Autodesk Inventor part; units mm, degrees
ref_plane "YZ Plane" through (0, 0, 0) normal (1, 0, 0) x (0, 1, 0)
ref_plane "XZ Plane" through (0, 0, 0) normal (0, 1, 0) x (-1, 0, 0)
ref_plane "XY Plane" through (0, 0, 0) normal (0, 0, 1) x (1, 0, 0)
ref_plane "Work Plane1" through (0, 0, 0) normal (0, 0, 1) x (1, 0, 0)
sketch "Sketch1" plane through (0, 0, 0) normal (0, 0, 1) x (1, 0, 0)
  line L0 (21.3787, 6.8051) -> (32.3787, 6.8051)
  line L1 (32.3787, 6.8051) -> (32.3787, -2.1949)
  line L2 (32.3787, -2.1949) -> (21.3787, -2.1949)
  line L3 (21.3787, -2.1949) -> (21.3787, 6.8051)
  point P0 (0, 0)
  dimension "d0" = 11
  dimension "d2" = 9
extrude "Extrusion1" add sketch "Sketch1" along normal blind 5
sketch "Sketch2" plane through (32.3787, -2.1949, 0) normal (1, 0, 0) x (0, 0, -1)
  circle A0 centre (-2.5, 4.5) radius 3.1
  point P0 (0, 2.1949)
  dimension "d5" = 6.2
extrude "Extrusion2" add sketch "Sketch2" along normal blind 4
sketch "Sketch3" plane through (36.3787, 2.3051, 2.5) normal (1, 0, 0) x (0, 0, -1)
  circle A0 centre (0, 0) radius 3.1
  circle A1 centre (0, 0) radius 1.75
  point P0 (2.5, -2.3051)
  dimension "d9" = 3.5
extrude "Extrusion3" cut sketch "Sketch3" against normal blind 7 contours A1
properties part number "nanopc_t4_headphone"
Geometry: final body of the model. Coordinates: model frame, mm. A direction names the side the tool comes from. Round coordinates to 2 decimals unless told otherwise and drop trailing zeros. Write each loop counter-clockwise with the first axis right and the second up, starting at its lowest first coordinate (ties: lowest second). Pieces come first, ordered by that corner, then holes. Notation, with made-up numbers: M -29,28.5 L 2,28.5 A21 cw 2,32.5 Z; hole C 6.25,33.25 d3. An arc over 180 degrees is marked long. Answer in a Markdown table with one row per item. Add a question column.
(1) Cut plane D-D, the plane y = 0. Return the cut outline in (x, z), then the cut area to 3 significant figures.
(2) Reachability of faces 1 (the face through (36.379, 1, 1)), 2 (the face through (27, 2, 0)), 3 (the face through (32.928, 0.753, 1.692)) from +Z, -Z, +X, -X, +Y, -Y: full face, straight path, thin tool, end or side. Return the list, or none.
(3) Contact query for flat-ended pins moving along their axis: pin 1 (0.7 mm diameter, centred on y = 3, z = 5.5, fed in from -X); pin 2 (4 mm diameter, centred on x = 31, y = 0.5, fed in from +Z); pin 3 (1.5 mm diameter, centred on x = 33.5, z = 4.5, fed in from -Y). Output: stop coordinate, or through.
(4) Draft query along Y for faces 4 (the face through (34.351, 1.374, -0.457)), 5 (the face through (29.379, 2, 3)), 6 (the face through (27, 2, 5)). Return one class per face: pulls with the +Y half, pulls with the -Y half, needs draft (parallel to the pull), parting line crosses it, or undercut.
(5) Cut plane C-C, the plane x = 34.25. Return the cut outline in (y, z).
(6) Cut plane A-A, the plane z = 2.5. Return the cut outline in (x, y), then the cut area to 3 significant figures.
(7) Ray query, L1, parallel to Y at x = 32, z = 2.5; L2, parallel to Y at x = 33.5, z = 2.5; L3, parallel to Z at x = 24, y = 5. Return the intervals inside material, ascending.
(8) Cut plane B-B, the plane y = 1.25. Return the cut outline in (x, z), then the cut area to 3 significant figures.
Established:
| question | item | result |
|---|---|---|
| 1 | outline | M 21.38,0 L 32.38,0 L 32.38,0.43 L 36.38,0.43 L 36.38,4.57 L 32.38,4.57 L 32.38,5 L 21.38,5 Z |
| 1 | area | 71.6 mm² |
| 2 | face 1 | +Z, -Z, +X, +Y, -Y |
| 2 | face 2 | -Z, -X, +Y, -Y |
| 2 | face 3 | +X |
| 3 | pin 1 | x = 32.38 |
| 3 | pin 2 | z = 5.58 |
| 3 | pin 3 | y = -0.53 |
| 4 | face 4 | parting line crosses it |
| 4 | face 5 | undercut |
| 4 | face 6 | needs draft |
| 5 | outline | C 2.31,2.5 d6.2; hole C 2.31,2.5 d3.5 |
| 6 | outline | M 21.38,-2.19 L 32.38,-2.19 L 32.38,-0.79 L 36.38,-0.79 L 36.38,0.56 L 29.38,0.56 L 29.38,4.06 L 36.38,4.06 L 36.38,5.41 L 32.38,5.41 L 32.38,6.81 L 21.38,6.81 Z |
| 6 | area | 99.3 mm² |
| 7 | L1 | -2.19 to 0.56, 4.06 to 6.81 |
| 7 | L2 | -0.79 to 0.56, 4.06 to 5.41 |
| 7 | L3 | 0 to 5 |
| 8 | outline | M 21.38,0 L 32.38,0 L 32.38,-0.41 L 36.38,-0.41 L 36.38,1.1 L 29.38,1.1 L 29.38,3.9 L 36.38,3.9 L 36.38,5.41 L 32.38,5.41 L 32.38,5 L 21.38,5 Z |
| 8 | area | 58.8 mm² |
